from build123d import *

# Parameters (mm, degrees)
SKETCH1_W           = 508
SKETCH1_H           = 254
BOSS_EXTRUDE1_DEPTH = 6.35
SKETCH3_R           = 11.938
SKETCH3_R_2         = 6
SKETCH3_R_3         = 14
CUT_EXTRUDE2_DEPTH  = 568.996762755
FILLET1_R           = 12.7
SKETCH4_R           = 2.0701
SKETCH4_R_2         = 2.4892
CUT_EXTRUDE3_DEPTH  = 568.996762755


with BuildPart() as part:
    # Sketch1 → Boss-Extrude1 (new body)
    with BuildSketch(Plane.XY):
        with Locations((254, 127)):
            Rectangle(SKETCH1_W, SKETCH1_H)
    extrude(amount=BOSS_EXTRUDE1_DEPTH)

    # Sketch3 → Cut-Extrude2 (cut, through all)
    with BuildSketch(Plane(origin=(0, 0, 0), x_dir=(-1, 0, 0), z_dir=(0, 0, -1))):
        with Locations((-158.75, 88.9)):
            Circle(SKETCH3_R)
        with Locations((-222.25, 88.9)):
            Circle(SKETCH3_R)
        with Locations((-158.75, 50.8)):
            Circle(SKETCH3_R)
        with Locations((-222.25, 50.8)):
            Circle(SKETCH3_R)
        with Locations((-222.25, 127)):
            Circle(SKETCH3_R)
        with Locations((-285.75, 127)):
            Circle(SKETCH3_R)
        with Locations((-285.75, 88.9)):
            Circle(SKETCH3_R)
        with Locations((-285.75, 50.8)):
            Circle(SKETCH3_R)
        with Locations((-254, 203.2)):
            Circle(SKETCH3_R_2)
        with Locations((-190.5, 203.2)):
            Circle(SKETCH3_R_2)
        with Locations((-158.75, 127)):
            Circle(SKETCH3_R)
        with Locations((-190.5, 165.1)):
            Circle(SKETCH3_R)
        with Locations((-254, 165.1)):
            Circle(SKETCH3_R)
        with Locations((-88.9, 165.1)):
            Circle(SKETCH3_R_3)
    extrude(amount=-CUT_EXTRUDE2_DEPTH, mode=Mode.SUBTRACT)

    # Fillet1
    fillet1_edges = [part.edges().sort_by_distance(p)[0] for p in [
        (0, 254, 3.175),
        (508, 254, 3.175),
        (508, 0, 3.175),
        (0, 0, 3.175),
    ]]
    fillet(fillet1_edges, radius=FILLET1_R)

    # Sketch4 → Cut-Extrude3 (cut, through all)
    with BuildSketch(Plane(origin=(0, 0, 0), x_dir=(-1, 0, 0), z_dir=(0, 0, -1))):
        with Locations((-495.320545376, 241.3)):
            Circle(SKETCH4_R)
        with Locations((-469.920545376, 241.3)):
            Circle(SKETCH4_R)
        with Locations((-495.320545376, 215.9)):
            Circle(SKETCH4_R_2)
        with Locations((-495.320545376, 203.2)):
            Circle(SKETCH4_R_2)
        with Locations(Location((-469.920545376, 12.7, 0), (0, 0, 180))):
            Circle(SKETCH4_R)
        with Locations(Location((-495.320545376, 50.8, 0), (0, 0, 180))):
            Circle(SKETCH4_R_2)
        with Locations(Location((-495.320545376, 38.1, 0), (0, 0, 180))):
            Circle(SKETCH4_R_2)
        with Locations(Location((-495.320545376, 12.7, 0), (0, 0, 180))):
            Circle(SKETCH4_R)
    extrude(amount=-CUT_EXTRUDE3_DEPTH, mode=Mode.SUBTRACT)


solid = part.part
Could you check a few things on this model? Use its own coordinates, in mm. Give positions to 0.01 mm unless a question says otherwise; leave off trailing zeros. Order: outer loops, then holes, each group sorted by start corner. A loop starts at its lowest first (then second) coordinate and runs counter-clockwise, first axis right, second up.
1. Suppose I cut it at C-C (y = 88.9). Write out the boundary of the cut face in (x, z).
Answers below:
outline: (0, 0) - (146.81, 0) - (146.81, 6.35) - (0, 6.35) - close; (170.69, 0) - (210.31, 0) - (210.31, 6.35) - (170.69, 6.35) - close; (234.19, 0) - (273.81, 0) - (273.81, 6.35) - (234.19, 6.35) - close; (297.69, 0) - (508, 0) - (508, 6.35) - (297.69, 6.35) - close
2. I need wall thicknesses on L1, parallel to Y at x = 222.25, z = 2.25; L2, parallel to Y at x = 254, z = 3; L3, parallel to X at y = 117, z = 6. Which ranges of each line are inside material? Lowest first, please.
Answers below:
L1: y = 0 to 38.86, 62.74 to 76.96, 100.84 to 115.06, 138.94 to 254
L2: y = 0 to 153.16, 177.04 to 197.2, 209.2 to 254
L3: x = 0 to 152.23, 165.27 to 215.73, 228.77 to 279.23, 292.27 to 508
3. Suppose I cut it at A-A (z = 4). State how many separate pieces and enclosed holes the cut face has, plus the area to 3 significant figures.
Answers below:
separate pieces: 1
enclosed holes: 22
area: 123,000 mm2
4. Suppose I cut it at B-B (x = 222.25). Write out the boundary of the cut face in (y, z).
Answers below:
outline: (0, 0) - (38.86, 0) - (38.86, 6.35) - (0, 6.35) - close; (62.74, 0) - (76.96, 0) - (76.96, 6.35) - (62.74, 6.35) - close; (100.84, 0) - (115.06, 0) - (115.06, 6.35) - (100.84, 6.35) - close; (138.94, 0) - (254, 0) - (254, 6.35) - (138.94, 6.35) - close
5. Thinking about a two-plate mould opening in Y: for faces 1 (the flat face through (250, 129, 0)), 2 (the cylindrical face through (3.62, 250.18, 3.22)), 3 (the cylindrical face through (102.886, 165.716, 3.131)), which applies, +Y half, -Y half, draft (parallel to the pull), parting line (faces both ways), or undercut?
Answers below:
face 1: draft
face 2: +Y half
face 3: undercut
6. Suppose I cut it at D-D (x = 88.9). Write out the boundary of the cut face in (y, z), plus the area to 3 significant figures.
Answers below:
outline: (0, 0) - (151.1, 0) - (151.1, 6.35) - (0, 6.35) - close; (179.1, 0) - (254, 0) - (254, 6.35) - (179.1, 6.35) - close
area: 1,440 mm2
7. For pin 1 (3.5 mm diameter, centred on x = 469.92, y = 12.7, fed in from -Z), with a flat end and sliding along its axis, tell me the tip position at first contact or that it passes through.
Answers below:
pin 1: passes through
